```python
from build123d import *

# Parameters (mm, degrees)
SKETCH1_R               = 12.7
SKETCH1_R_2             = 11.90625
BOSS_EXTRUDE1_DEPTH     = 2443.872227937
SKETCH4_W               = 2.75
SKETCH4_H               = 12.7
SKETCH12_W              = 2.75
SKETCH12_H              = 12.7
SKETCH13_R              = 2.750000003
CUT_EXTRUDE1_DEPTH      = 13.7000001
CUT_EXTRUDE1_DEPTH_BACK = 13.7000001


with BuildPart() as part:
    # Sketch1 → Boss-Extrude1 (new body)
    with BuildSketch(Plane.XY):
        Circle(SKETCH1_R)
        Circle(SKETCH1_R_2, mode=Mode.SUBTRACT)
    extrude(amount=BOSS_EXTRUDE1_DEPTH)

    # Sketch4 → M5 Clearance Hole1 (revolve, cut)
    with BuildSketch(Plane(origin=(0, 0, 2436.622227937), x_dir=(0, 0, -1), z_dir=(1, 0, 0))):
        with Locations((1.375, 6.35)):
            Rectangle(SKETCH4_W, SKETCH4_H)
    m5_clearance_hole1 = revolve(axis=Axis((0, -6.35, 2436.622227937), (0, 1, 0)), mode=Mode.SUBTRACT)

    # Mirror1: M5 Clearance Hole1 across plane
    add(m5_clearance_hole1.mirror(Plane.ZX), mode=Mode.SUBTRACT)

    # Sketch12 → M5 Clearance Hole3 (revolve, cut)
    with BuildSketch(Plane(origin=(0, 0, 15), x_dir=(0, 0, 1), z_dir=(0, 1, 0))):
        with Locations((1.375, 6.35)):
            Rectangle(SKETCH12_W, SKETCH12_H)
    m5_clearance_hole3 = revolve(axis=Axis((-6.35, 0, 15), (1, 0, 0)), mode=Mode.SUBTRACT)

    # Mirror3: M5 Clearance Hole3 across plane
    add(m5_clearance_hole3.mirror(Plane(origin=(0, 0, 0), x_dir=(0, 0, 1), z_dir=(1, 0, 0))), mode=Mode.SUBTRACT)

    # Sketch13 → Cut-Extrude1 (cut, two sides)
    with BuildSketch(Plane(origin=(0, 0, 0), x_dir=(1, 0, 0), z_dir=(0, 1, 0))) as cut_extrude1_sk:
        with Locations((-0.739798723, -1718.754532743)):
            Circle(SKETCH13_R)
    extrude(amount=CUT_EXTRUDE1_DEPTH, mode=Mode.SUBTRACT)
    extrude(cut_extrude1_sk.sketch, amount=-CUT_EXTRUDE1_DEPTH_BACK, mode=Mode.SUBTRACT)


solid = part.part
```
Input: part model. Units: mm. Frame: model coordinates. Round coordinates to 2 decimals unless told otherwise and drop trailing zeros. Write each loop counter-clockwise with the first axis right and the second up, starting at its lowest first coordinate (ties: lowest second). Pieces come first, ordered by that corner, then holes. Notation, with made-up numbers: (28.25, -0.75) - (57.25, -0.75) arc R21 ccw to (57.25, 28.25) - close; hole circle Ø10 at (23.25, 46). An arc over 180 degrees is marked (long way). Write item = value, one per line.
(1) Contact query for flat-ended pins moving along their axis: pin 1 Ø7 at (x, z) = (0, 2436.62) entering from +Y; pin 2 Ø3 at (y, z) = (-4.5, 323) entering from +X; pin 3 Ø4 at (x, z) = (8, 501.5) entering from +Y; pin 4 Ø5 at (x, z) = (-8.5, 877.5) entering from -Y. Output: stop coordinate, or through.
Geometry check:
pin_1 = 12.7
pin_2 = 12.34
pin_3 = 11.19
pin_4 = -11.19
(2) Section query B-B on z = 1658.5. Output: boundary loops of the cut face in (x, y).
Geometry check:
outline = circle Ø25.4 at (0, 0); hole circle Ø23.81 at (0, 0)
(3) Material intervals for probe 1 along Z at (x, y) = (0, 12); probe 2 along Y at (x, z) = (4, 833.5), sorted ascending.
Geometry check:
probe_1 = 0 to 1716.11, 1721.4 to 2433.87, 2439.37 to 2443.87
probe_2 = -12.05 to -11.21, 11.21 to 12.05
(4) Section query A-A on y = 7.25. Output: boundary loops of the cut face in (x, z), then the cut area to 3 significant figures.
Geometry check:
outline = (-10.43, 0) - (-9.44, 0) - (-9.44, 2443.87) - (-10.43, 2443.87) - close; (9.44, 0) - (10.43, 0) - (10.43, 2443.87) - (9.44, 2443.87) - close
area = 4,800 mm^2
